Autodesk Inventor part; units mm, degrees
ref_plane "Work Plane2" through (36.5, 0, 0) normal (1, 0, 0) x (0, 1, 0)
ref_plane "Work Plane3" through (0, 93, 0) normal (0, 1, 0) x (1, 0, 0)
ref_plane "Work Plane5" through (0, 32, 0) normal (0, 1, 0) x (1, 0, 0)
sketch "Sketch1" plane through (0, 0, 0) normal (0, 1, 0) x (-1, 0, 0)
  circle A0 centre (0, 0) radius 36.5
  circle A1 centre (0, 0) radius 35
  dimension "d0" = 73
  dimension "d1" = 70
extrude "Extrusion1" add sketch "Sketch1" along normal blind 3 contours A0 | A1
extrude "Extrusion2" add sketch "Sketch1" along normal blind 120
sketch "Sketch2" plane through (0, 3, 0) normal (0, 1, 0) x (1, 0, 0)
  circle A0 centre (0, 0) radius 35
  line L0 (-24.7487, -24.7487) -> (24.7487, -24.7487)
  line L1 (24.7487, -24.7487) -> (24.7487, 24.7487)
  line L2 (24.7487, 24.7487) -> (-24.7487, 24.7487)
  line L3 (-24.7487, 24.7487) -> (-24.7487, -24.7487)
  line L4 (-24.7487, -24.7487) -> (24.7487, 24.7487) construction
  line L5 (24.7487, -24.7487) -> (-24.7487, 24.7487) construction
extrude "Extrusion3" add sketch "Sketch2" along normal blind 2 contours L1 L0 L3 L2
sketch "Sketch3" plane through (0, 5, 0) normal (0, 1, 0) x (1, 0, 0)
  line L0 (21.1, -23.1) -> (-21.1, -23.1)
  line L1 (-23.1, -21.1) -> (-23.1, 21.1)
  line L2 (-21.1, 23.1) -> (21.1, 23.1)
  line L3 (23.1, 21.1) -> (23.1, -21.1)
  line L4 (23.1, -23.1) -> (-23.1, 23.1) construction
  line L5 (-23.1, -23.1) -> (23.1, 23.1) construction
  arc A0 (-23.1, -21.1) -> (-21.1, -23.1) centre (-21.1, -21.1) ccw
  arc A1 (21.1, -23.1) -> (23.1, -21.1) centre (21.1, -21.1) ccw
  arc A2 (23.1, 21.1) -> (21.1, 23.1) centre (21.1, 21.1) ccw
  arc A3 (-21.1, 23.1) -> (-23.1, 21.1) centre (-21.1, 21.1) ccw
  point P0 (0, 0)
  dimension "d11" = 46.2
  dimension "d12" = 46.2
  dimension "d13" = 2
extrude "Extrusion4" cut sketch "Sketch3" against normal blind 2
sketch "Sketch4" plane through (0, 0, 0) normal (1, 0, 0) x (0, 1, 0)
  line L0 (120, 35) -> (120, -35)
  line L1 (120, 0) -> (120, -19.5)
  line L2 (120, -19.5) -> (120, -27)
  circle A0 centre (120, -27) radius 9
  point P0 (0, 0)
  dimension "d16" = 19.5
  dimension "d17" = 7.5
  dimension "d18" = 18
extrude "Extrusion5" cut sketch "Sketch4" along normal through all
sketch "Sketch5" plane through (0, 0, 0) normal (0, -1, 0) x (1, 0, 0)
  line L0 (5, -36.1559) -> (5, -42.4125)
  line L1 (5, -42.4125) -> (-5, -42.4125)
  line L2 (-5, -42.4125) -> (-5, -36.1559)
  line L3 (-5, -30.5875) -> (5, -42.4125) construction
  line L4 (5, -30.5875) -> (-5, -42.4125) construction
  circle A0 centre (0, 0) radius 36.5
  line L5 (8, -35.6125) -> (8, -42.4125)
  line L6 (8, -42.4125) -> (-8, -42.4125)
  line L7 (-8, -42.4125) -> (-8, -35.6125)
  line L8 (-8, -30.5875) -> (8, -42.4125) construction
  line L9 (8, -30.5875) -> (-8, -42.4125) construction
  circle A1 centre (0, 0) radius 36.5
  arc A2 (5, -36.1675) -> (4.9876, -36.1576) centre (0, -42.4125) ccw
  arc A3 (-4.9876, -36.1576) -> (-5, -36.1675) centre (0, -42.4125) ccw
  arc A4 (-8, -42.4125) -> (8, -42.4125) centre (0, -42.4125) ccw
  arc A5 (-5, -42.4125) -> (5, -42.4125) centre (0, -42.4125) ccw
  point P0 (0, -36.5)
  dimension "d21" = 10
  dimension "d22" = 36.5
  dimension "d23" = 16
extrude "Extrusion6" add sketch "Sketch5" against normal blind 6 contours A0 L5 L6 L0 | L6 A4 A5 | L6 L7 A0 L2
ref_plane "Work Plane2" through (36.5, 0, 0) normal (1, 0, 0) x (0, 1, 0)
sketch "Sketch8" plane through (36.5, 0, 0) normal (1, 0, 0) x (0, 1, 0)
  line L0 (8.45, 4.25) -> (21.55, 4.25)
  line L1 (21.55, 4.25) -> (21.55, -4.25)
  line L2 (21.55, -4.25) -> (8.45, -4.25)
  line L3 (8.45, -4.25) -> (8.45, 4.25)
  line L4 (8.45, 4.25) -> (21.55, -4.25) construction
  line L5 (21.55, 4.25) -> (8.45, -4.25) construction
  line L6 (7.5, 5.25) -> (22.5, 5.25)
  line L7 (22.5, 5.25) -> (22.5, -5.25)
  line L8 (22.5, -5.25) -> (7.5, -5.25)
  line L9 (7.5, -5.25) -> (7.5, 5.25)
  line L10 (7.5, 5.25) -> (22.5, -5.25) construction
  line L11 (22.5, 5.25) -> (7.5, -5.25) construction
  point P0 (0, 0)
  point P1 (15, 0)
  dimension "d38" = 13.1
  dimension "d39" = 8.5
  dimension "d40" = 0
  dimension "d41" = 15
  dimension "d42" = 10.5
  dimension "d43" = 15
extrude "Extrusion9" cut sketch "Sketch8" against normal blind 3 contours L0 L1 L2 L3
extrude "Extrusion10" cut sketch "Sketch8" against normal blind 1
ref_plane "Work Plane3" through (0, 93, 0) normal (0, 1, 0) x (1, 0, 0)
ref_plane "Work Plane5" through (0, 32, 0) normal (0, 1, 0) x (1, 0, 0)
sketch "Sketch13" plane through (0, 32, 0) normal (0, 1, 0) x (1, 0, 0)
  circle A0 centre (0, 0) radius 20
  line L0 (24.7487, 24.7487) -> (-24.7487, 24.7487)
  circle A1 centre (0, 0) radius 35
  dimension "d61" = 40
extrude "Extrusion14" add sketch "Sketch13" along normal blind 3
sketch "Sketch15" plane through (0, 32, 0) normal (0, 1, 0) x (1, 0, 0)
  circle A0 centre (0, 0) radius 61.7615
extrude "Extrusion16" cut sketch "Sketch15" along normal through all
sketch "Sketch16" plane through (0, 32, 0) normal (0, 1, 0) x (1, 0, 0)
  circle A0 centre (0, 0) radius 36.5
  circle A1 centre (0, 0) radius 38
  dimension "d68" = 76
  dimension "d69" = 73
extrude "Extrusion17" add sketch "Sketch16" along normal blind 10 and the other way blind 5
properties part number "bottom bottom"
Check sheet for the modelled part. Datum: model origin and axes. Units: mm. A direction names the side the tool comes from. Coordinates: 2 decimals unless noted, no trailing zeros. Order: outer loops, then holes, each group sorted by start corner. A loop starts at its lowest first (then second) coordinate and runs counter-clockwise, first axis right, second up. Notation, with made-up numbers: (36, -8) -> (64, -8) arc R25 cw to (64, 27) -> close; hole circle Ø1 at (41.25, -34.75). An arc over 180 degrees is marked (long way). Write item = value, one per line. Start each with the question number.
1) Cross-section at B-B (x = 0). Enter the section's corners in (y, z).
2) Cross-section at C-C (y = 12). Enter the section's corners in (x, z), then the cut area to 3 significant figures.
3) Access from +Z, -Z, +X, -X, +Y, -Y to the whole of each face (thin tool, end or side, straight path). Record for faces 1 (the cylindrical face through (-7.912, 36.93, -35.632)), 2 (the cylindrical face through (-0.11, 2.96, -47.41)), 3 (the flat face through (5, 3, -39)).
4) Cross-section at D-D (y = 38). Enter the section's corners in (x, z), then the cut area to 3 significant figures.
5) Mould release check, pull along X, two halves, no side actions. Record for faces 4 (the flat face through (-8, 3, -39)), 5 (the flat face through (8, 3, -39)), 6 (the flat face through (0, 4, 24.749)): +X half, -X half, draft (parallel to the pull), parting line (faces both ways), or undercut.
6) Go/stop test with flat-tipped pins: P1, Ø6, axis at x = -30, y = 37, coming from the +Z side; P2, Ø4, axis at x = -22.5, y = 33.5, coming from the -Z side; P3, Ø5, axis at x = 5.5, z = -31.5, coming from the +Y side. Record where each tip stops, or that it passes through.
7) Material ranges on L1, parallel to X at y = 39, z = 0; L2, parallel to Z at x = 0, y = 11, recorded low to high.
Ans:
q1.outline = (0, -50.41) -> (6, -50.41) -> (6, -47.41) -> (0, -47.41) -> close; (0, -36.5) -> (27, -36.5) -> (27, -38) -> (42, -38) -> (42, -36.5) -> (32, -36.5) -> (32, -35) -> (3, -35) -> (3, -24.75) -> (5, -24.75) -> (5, -23.1) -> (3, -23.1) -> (3, 23.1) -> (5, 23.1) -> (5, 24.75) -> (3, 24.75) -> (3, 35) -> (32, 35) -> (32, 36.5) -> (42, 36.5) -> (42, 38) -> (27, 38) -> (27, 36.5) -> (0, 36.5) -> close
q2.outline = (34.74, -4.25) arc R35 cw (long way) to (34.74, 4.25) -> (35.5, 4.25) -> (35.5, 5.25) -> (36.12, 5.25) arc R36.5 ccw (long way) to (36.12, -5.25) -> (35.5, -5.25) -> (35.5, -4.25) -> close
q2.area = 323 mm²
q3.face_1 = +Y
q3.face_2 = +Y, -Y
q3.face_3 = -Y
q4.outline = circle Ø76 at (0, 0); hole circle Ø73 at (0, 0)
q4.area = 351 mm²
q5.face_4 = -X half
q5.face_5 = +X half
q5.face_6 = undercut
q6.P1 = 26.74
q6.P2 = -32
q6.P3 = 3
q7.L1 = -38 to -36.5, 36.5 to 38
q7.L2 = -36.5 to -35, 35 to 36.5
